Autodesk Inventor part; units mm, degrees
ref_plane "YZ Plane" through (0, 0, 0) normal (1, 0, 0) x (0, 1, 0)
ref_plane "XZ Plane" through (0, 0, 0) normal (0, 1, 0) x (-1, 0, 0)
ref_plane "XY Plane" through (0, 0, 0) normal (0, 0, 1) x (1, 0, 0)
sketch "Sketch1" plane through (0, 0, 0) normal (0, 0, 1) x (1, 0, 0)
  line L0 (0, 0) -> (0, 15)
  line L1 (0, 15) -> (15, 15)
  line L2 (15, 15) -> (15, 60)
  line L3 (15, 60) -> (-65, 60)
  line L4 (-65, 60) -> (-65, 0)
  line L5 (-65, 0) -> (0, 0)
  line L6 (-36.8, 25) -> (-36.8, 20) construction
  line L7 (-38.4, 25) -> (-38.4, 20)
  line L8 (-35.2, 20) -> (-35.2, 25)
  arc A0 (-35.2, 25) -> (-38.4, 25) centre (-36.8, 25) ccw
  arc A1 (-38.4, 20) -> (-35.2, 20) centre (-36.8, 20) ccw
  line L9 (-5.8, 25) -> (-5.8, 20) construction
  line L10 (-7.4, 25) -> (-7.4, 20)
  line L11 (-4.2, 20) -> (-4.2, 25)
  arc A2 (-4.2, 25) -> (-7.4, 25) centre (-5.8, 25) ccw
  arc A3 (-7.4, 20) -> (-4.2, 20) centre (-5.8, 20) ccw
  line L12 (-5.8, 56) -> (-5.8, 51) construction
  line L13 (-7.4, 56) -> (-7.4, 51)
  line L14 (-4.2, 51) -> (-4.2, 56)
  arc A4 (-4.2, 56) -> (-7.4, 56) centre (-5.8, 56) ccw
  arc A5 (-7.4, 51) -> (-4.2, 51) centre (-5.8, 51) ccw
  line L15 (-36.8, 56) -> (-36.8, 51) construction
  line L16 (-38.4, 56) -> (-38.4, 51)
  line L17 (-35.2, 51) -> (-35.2, 56)
  arc A6 (-35.2, 56) -> (-38.4, 56) centre (-36.8, 56) ccw
  arc A7 (-38.4, 51) -> (-35.2, 51) centre (-36.8, 51) ccw
  line L18 (-21.3, 40.5) -> (-21.3, 35.5) construction
  line L19 (-32.8, 40.5) -> (-32.8, 35.5)
  line L20 (-9.8, 35.5) -> (-9.8, 40.5)
  arc A8 (-9.8, 40.5) -> (-32.8, 40.5) centre (-21.3, 40.5) ccw
  arc A9 (-32.8, 35.5) -> (-9.8, 35.5) centre (-21.3, 35.5) ccw
  line L21 (-41.8, 60) -> (-41.8, 41)
  line L22 (-41.8, 41) -> (-55, 41)
  line L23 (-55, 41) -> (-65, 31)
  point P0 (-36.8, 22.5)
  point P1 (-5.8, 22.5)
  point P2 (-5.8, 53.5)
  point P3 (-36.8, 53.5)
  point P4 (-21.3, 38)
  dimension "d0" = 15
  dimension "d57" = 3.2
  dimension "d58" = 31
  dimension "d59" = 31
  dimension "d60" = 36.3
  dimension "d61" = 11.5
  dimension "d62" = 5
  dimension "d63" = 15.5
  dimension "d64" = 15.5
  dimension "d65" = 60
  dimension "d66" = 80
  dimension "d67" = 38
  dimension "d68" = 45
  dimension "d69" = 31
  dimension "d70" = 19
  dimension "d71" = 5
extrude "Extrusion1" add sketch "Sketch1" along normal blind 4 contours L5 L4 L23 L22 L21 L3 L2 L1 L0
sketch "Sketch2" plane through (0, 0, 0) normal (0, 0, -1) x (-1, 0, 0)
  line L0 (0, 15) -> (-15, 15)
  line L1 (0, 0) -> (0, 15)
  line L2 (65, 0) -> (0, 0)
  line L3 (65, 31) -> (65, 0)
  line L4 (-15, 60) -> (41.8, 60)
  line L5 (-15, 15) -> (-15, 60)
  line L6 (0, 15) -> (65, 15)
  line L7 (65, 31) -> (65, 0)
  line L8 (0, 15) -> (-15, 15)
  line L9 (0, 15) -> (0, 60)
  line L10 (-15, 60) -> (41.8, 60)
  line L11 (55, 41) -> (65, 31)
  line L12 (41.8, 41) -> (55, 41)
  line L13 (41.8, 60) -> (41.8, 41)
  point P0 (65, 60)
  point P1 (0, 60)
extrude "Extrusion2" add sketch "Sketch2" along normal blind 3 contours L6 L3 L2 L1 | L0 L5 L4 L9
sketch "Sketch3" plane through (0, 0, 4) normal (0, 0, 1) x (1, 0, 0)
  line L0 (-65, 31) -> (-65, 0)
  line L1 (-65, 0) -> (0, 0)
  line L2 (0, 0) -> (0, 15)
  line L3 (0, 15) -> (15, 15)
  line L4 (15, 15) -> (15, 60)
  line L5 (15, 60) -> (-41.8, 60)
  line L6 (-65, 0) -> (-65, 15)
  line L7 (0, 60) -> (15, 60)
  line L8 (-41.8, 60) -> (-41.8, 41)
  line L9 (-41.8, 41) -> (-55, 41)
  line L10 (-55, 41) -> (-65, 31)
  point P0 (-10, 7.5)
  point P1 (-55, 7.5)
  point P2 (7.5, 25)
  point P3 (7.5, 50)
  point P4 (0, 7.5)
  point P5 (-65, 7.5)
  point P6 (7.5, 15)
  point P7 (7.5, 60)
  dimension "d18" = 10
  dimension "d19" = 10
  dimension "d20" = 10
  dimension "d21" = 10
hole "Hole1" at (-10, 7.5, 4) at (-55, 7.5, 4) at (7.5, 25, 4) at (7.5, 50, 4) direction (0, 0, -1) diameter 3.6 end through all counterbore diameter 6.5 counterbore depth 3.4
sketch "Sketch8" plane through (0, 0, 0) normal (0, 0, -1) x (-1, 0, 0)
  line L0 (0, 15) -> (65, 15)
  line L1 (65, 31) -> (65, 15)
  line L2 (55, 41) -> (65, 31)
  line L3 (41.8, 41) -> (55, 41)
  line L4 (41.8, 60) -> (41.8, 41)
  line L5 (0, 60) -> (41.8, 60)
  line L6 (0, 60) -> (0, 15)
  arc A0 (32.8, 40.5) -> (9.8, 40.5) centre (21.3, 40.5) ccw
  line L7 (32.8, 35.5) -> (32.8, 40.5)
  arc A1 (9.8, 35.5) -> (32.8, 35.5) centre (21.3, 35.5) ccw
  line L8 (9.8, 40.5) -> (9.8, 35.5)
  arc A2 (38.4, 56) -> (35.2, 56) centre (36.8, 56) ccw
  line L9 (38.4, 51) -> (38.4, 56)
  arc A3 (35.2, 51) -> (38.4, 51) centre (36.8, 51) ccw
  line L10 (35.2, 56) -> (35.2, 51)
  arc A4 (7.4, 56) -> (4.2, 56) centre (5.8, 56) ccw
  line L11 (7.4, 51) -> (7.4, 56)
  arc A5 (4.2, 51) -> (7.4, 51) centre (5.8, 51) ccw
  line L12 (4.2, 56) -> (4.2, 51)
  arc A6 (7.4, 25) -> (4.2, 25) centre (5.8, 25) ccw
  line L13 (7.4, 20) -> (7.4, 25)
  arc A7 (4.2, 20) -> (7.4, 20) centre (5.8, 20) ccw
  line L14 (4.2, 25) -> (4.2, 20)
  arc A8 (38.4, 25) -> (35.2, 25) centre (36.8, 25) ccw
  line L15 (38.4, 20) -> (38.4, 25)
  arc A9 (35.2, 20) -> (38.4, 20) centre (36.8, 20) ccw
  line L16 (35.2, 25) -> (35.2, 20)
  line L17 (41.8, 41) -> (55, 41)
  line L18 (41.8, 41) -> (41.8, 15)
  point P0 (0, 0)
extrude "Extrusion5" add sketch "Sketch8" along normal blind 21 contours L18 L3 L2 L1 L0
sketch "Sketch9" plane through (-41.8, 41, 4) normal (-1, 0, 0) x (0, 0, 1)
  line L0 (-4, 19) -> (-4, 0)
  line L1 (-4, 0) -> (0, 0)
  line L2 (0, 19) -> (0, 0)
  line L3 (-4, 19) -> (0, 19)
  line L4 (-4, 0) -> (0, 0)
  line L5 (-4, 0) -> (-28, 0)
  line L6 (-28, 0) -> (-28, 3)
  line L7 (-28, 3) -> (-9, 19)
  line L8 (-9, 19) -> (-4, 19)
  line L9 (0, 19) -> (-7, 19)
  line L10 (-21.4252, 2) -> (-7, 14.1475)
  line L11 (-7, 14.1475) -> (-7, 2)
  line L12 (-7, 2) -> (-21.4252, 2)
  point P0 (-4, -41)
  dimension "d74" = 24
  dimension "d75" = 3
  dimension "d76" = 5
  dimension "d77" = 5
  dimension "d78" = 3
  dimension "d79" = 2
extrude "Extrusion6" add sketch "Sketch9" along normal blind 5
sketch "Sketch10" plane through (0, 0, 0) normal (0, 0, -1) x (-1, 0, 0)
  line L0 (41.8, 60) -> (41.8, 15)
  line L1 (0, 60) -> (41.8, 60)
  line L2 (0, 60) -> (0, 15)
  line L3 (0, 15) -> (41.8, 15)
  arc A0 (32.8, 40.5) -> (9.8, 40.5) centre (21.3, 40.5) ccw
  line L4 (32.8, 35.5) -> (32.8, 40.5)
  arc A1 (9.8, 35.5) -> (32.8, 35.5) centre (21.3, 35.5) ccw
  line L5 (9.8, 40.5) -> (9.8, 35.5)
  arc A2 (38.4, 56) -> (35.2, 56) centre (36.8, 56) ccw
  line L6 (38.4, 51) -> (38.4, 56)
  arc A3 (35.2, 51) -> (38.4, 51) centre (36.8, 51) ccw
  line L7 (35.2, 56) -> (35.2, 51)
  arc A4 (7.4, 56) -> (4.2, 56) centre (5.8, 56) ccw
  line L8 (7.4, 51) -> (7.4, 56)
  arc A5 (4.2, 51) -> (7.4, 51) centre (5.8, 51) ccw
  line L9 (4.2, 56) -> (4.2, 51)
  arc A6 (7.4, 25) -> (4.2, 25) centre (5.8, 25) ccw
  line L10 (7.4, 20) -> (7.4, 25)
  arc A7 (4.2, 20) -> (7.4, 20) centre (5.8, 20) ccw
  line L11 (4.2, 25) -> (4.2, 20)
  arc A8 (38.4, 25) -> (35.2, 25) centre (36.8, 25) ccw
  line L12 (38.4, 20) -> (38.4, 25)
  arc A9 (35.2, 20) -> (38.4, 20) centre (36.8, 20) ccw
  line L13 (35.2, 25) -> (35.2, 20)
  line L14 (36.8, 56) -> (36.8, 51) construction
  line L15 (40.05, 56) -> (40.05, 51)
  line L16 (33.55, 51) -> (33.55, 56)
  arc A10 (40.05, 56) -> (33.55, 56) centre (36.8, 56) ccw
  arc A11 (33.55, 51) -> (40.05, 51) centre (36.8, 51) ccw
  line L17 (5.8, 51) -> (5.8, 56) construction
  line L18 (2.55, 51) -> (2.55, 56)
  line L19 (9.05, 56) -> (9.05, 51)
  arc A12 (2.55, 51) -> (9.05, 51) centre (5.8, 51) ccw
  arc A13 (9.05, 56) -> (2.55, 56) centre (5.8, 56) ccw
  line L20 (5.8, 20) -> (5.8, 25) construction
  line L21 (2.55, 20) -> (2.55, 25)
  line L22 (9.05, 25) -> (9.05, 20)
  arc A14 (2.55, 20) -> (9.05, 20) centre (5.8, 20) ccw
  arc A15 (9.05, 25) -> (2.55, 25) centre (5.8, 25) ccw
  line L23 (36.8, 20) -> (36.8, 25) construction
  line L24 (40.05, 20) -> (40.05, 25)
  line L25 (33.55, 25) -> (33.55, 20)
  arc A16 (33.55, 20) -> (40.05, 20) centre (36.8, 20) ccw
  arc A17 (40.05, 25) -> (33.55, 25) centre (36.8, 25) ccw
  point P0 (0, 0)
  point P1 (36.8, 53.5)
  point P2 (5.8, 53.5)
  point P3 (5.8, 22.5)
  point P4 (36.8, 22.5)
  dimension "d82" = 6.5
extrude "Extrusion7" cut sketch "Sketch10" against normal blind 1.5 contours L15 A11 L16 A10 | L18 A13 L19 A12 | L21 A15 L22 A14 | A16 L25 A17 L24
properties part number "Alpha Motor Mount" material "ABS Plastic"
CAD build for the part. Positions are in the model's coordinates, mm. A direction names the side the tool comes from. Coordinates: 2 decimals unless noted, no trailing zeros. Write each loop counter-clockwise with the first axis right and the second up, starting at its lowest first coordinate (ties: lowest second). Pieces come first, ordered by that corner, then holes. Notation, with made-up numbers: (34.5, -35.5) -> (59.5, -35.5) arc R19 cw to (59.5, -3.5) -> close; hole circle Ø2 at (-17.5, 80.25). An arc over 180 degrees is marked (long way). Use CSV: the item, a comma, the result in double quotes. Start each with the question number.
Item 1: Wall check: probe 1 along Y at (x, z) = (7.5, 1.45); probe 2 along X at (y, z) = (25, -2); probe 3 along X at (y, z) = (50, -1.2). Give the ranges that are in metal, low to high.
Item 2: Band-saw the part on A-A, the plane y = 37.5. Write the cut outline in (x, z).
Item 3: Band-saw the part on D-D, the plane z = -13.5. Write the cut outline in (x, y), plus the area to 3 significant figures.
Item 4: Band-saw the part on C-C, the plane x = -21.3. Write the cut outline in (y, z), plus the area to 3 significant figures.
Item 5: Drop flat-ended pins along their axis: P1, Ø10, axis at x = -48, z = -16, coming from the -Y side; P2, Ø9.5, axis at y = 55, z = -8, coming from the -X side; P3, Ø12, axis at y = 53, z = -15, coming from the +X side. Give the stop position or say it passes through.
Item 6: Two-plate mould, pull along X, no slides. Class faces 5 (the flat face through (-9.8, 38, 2)), 6 (the flat face through (-60, 36, -8)), 7 (the flat face through (0, 7, 0)): +X half, -X half, draft (parallel to the pull), parting line (faces both ways), or undercut.
Item 7: Band-saw the part on B-B, the plane x = 7.5. Write the cut outline in (y, z).
Item 8: Tool access for faces 1 (the cylindrical face through (-36.87, 28.25, 0.74)), 2 (the flat face through (-8.6, 6.1, 0.6)), 3 (the cylindrical face through (-5.8, 57.6, 2.7)), 4 (the flat face through (7, 15, 0)): list every direction of +Z, -Z, +X, -X, +Y, -Y with a clear straight run to the whole face (end or side of a thin tool).
Response values:
1,probe 1,"y = 15 to 21.75, 28.25 to 46.75, 53.25 to 60"
1,probe 2,"x = -65 to -41.8, 0 to 5.7, 9.3 to 15"
1,probe 3,"x = -46.8 to -41.8, 0 to 5.7, 9.3 to 15"
2,outline,"(-58.5, -21) -> (-41.8, -21) -> (-41.8, 0) -> (-32.8, 0) -> (-32.8, 4) -> (-58.5, 4) -> close; (-9.8, 0) -> (0, 0) -> (0, -3) -> (15, -3) -> (15, 4) -> (-9.8, 4) -> close"
3,outline,"(-65, 15) -> (-41.8, 15) -> (-41.8, 43) -> (-46.8, 43) -> (-46.8, 41) -> (-55, 41) -> (-65, 31) -> close; (-46.8, 46.31) -> (-41.8, 46.31) -> (-41.8, 52.84) -> (-46.8, 52.84) -> close"
3,area,"596 mm2"
4,outline,"(0, -3) -> (15, -3) -> (15, 0) -> (24, 0) -> (24, 4) -> (0, 4) -> close; (52, 0) -> (60, 0) -> (60, 4) -> (52, 4) -> close"
4,area,"173 mm2"
5,P1,"stops at y = 15"
5,P2,"stops at x = -46.8"
5,P3,"stops at x = -41.8"
6,face 5,"undercut"
6,face 6,"-X half"
6,face 7,"+X half"
7,outline,"(15, -3) -> (23.2, -3) -> (23.2, 0.6) -> (21.75, 0.6) -> (21.75, 4) -> (15, 4) -> close; (26.8, -3) -> (48.2, -3) -> (48.2, 0.6) -> (46.75, 0.6) -> (46.75, 4) -> (28.25, 4) -> (28.25, 0.6) -> (26.8, 0.6) -> close; (51.8, -3) -> (60, -3) -> (60, 4) -> (53.25, 4) -> (53.25, 0.6) -> (51.8, 0.6) -> close"
8,face 1,"-Z"
8,face 2,"+Z"
8,face 3,"+Z, -Z"
8,face 4,"+Z, -Z, +X, -Y"
